Could you check a few things on this model? Use its own coordinates, in mm. Round coordinates to 2 decimals unless told otherwise and drop trailing zeros. Loops run counter-clockwise (first coordinate to the right, second up) from the corner with the lowest first, then second, coordinate; pieces in that order, holes last. Notation, with made-up numbers: (-14, 80.25) -> (15, 80.25) arc R23 cw to (15, 91.25) -> close; hole circle Ø4 at (28, 76.25). An arc over 180 degrees is marked (long way). Use CSV: the item, a comma, the result in double quotes. Start each with the question number.
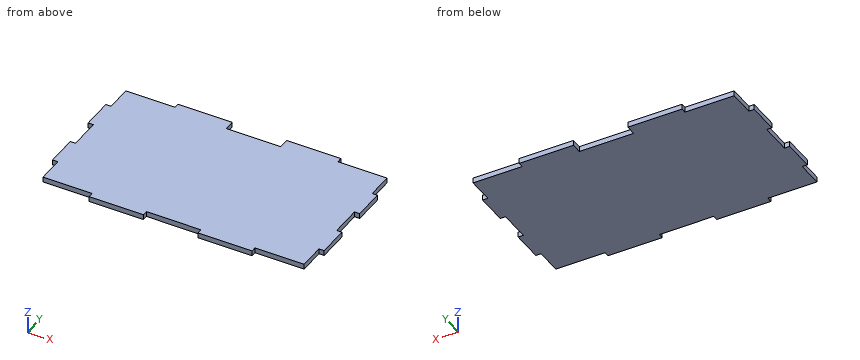
```python
from build123d import *

# Parameters (mm, degrees)
SALIENTE_EXTRUIR1_DEPTH = 5
CROQUIS2_W              = 52
CROQUIS2_H              = 5
CORTAR_EXTRUIR1_DEPTH   = 10


with BuildPart() as part:
    # Croquis1 → Saliente-Extruir1 (new body)
    with BuildSketch(Plane.XY):
        Polygon((52, 0), (104, 0), (104, 5), (156, 5), (156, 0), (208, 0), (208, 5), (255, 5), (255, 30), (260, 30), (260, 60), (255, 60), (255, 90), (260, 90), (260, 120), (255, 120), (255, 145), (208, 145), (208, 150), (156, 150), (156, 145), (104, 145), (104, 150), (52, 150), (52, 145), (5, 145), (5, 120), (0, 120), (0, 90), (5, 90), (5, 60), (0, 60), (0, 30), (5, 30), (5, 5), (52, 5), align=None)
    extrude(amount=SALIENTE_EXTRUIR1_DEPTH)

    # Croquis2 → Cortar-Extruir1 (cut)
    with BuildSketch(Plane.XY.offset(5)):
        with Locations((130, 142.5)):
            Rectangle(CROQUIS2_W, CROQUIS2_H)
    extrude(amount=-CORTAR_EXTRUIR1_DEPTH, mode=Mode.SUBTRACT)


solid = part.part
```
1. Will these pins go through, and if not, where does the flat tip stop? pin 1 (1.5 mm diameter, centred on x = 258, z = 3, fed in from +Y); pin 2 (2 mm diameter, centred on x = 145, y = 96, fed in from -Z); pin 3 (1.5 mm diameter, centred on x = 134.5, z = 2, fed in from +Y); pin 4 (2.5 mm diameter, centred on y = 2.5, z = 2, fed in from +X).
2. If I drill on L1, parallel to X at y = 143, z = 1.95; L2, parallel to Y at x = 140, z = 3.1; L3, parallel to X at y = 12, z = 4.6, over which ranges is the centre line in solid material (lowest first)?
3. Suppose I cut it at B-B (y = 16.5). List the corners of the cut face in (x, z) for me, then the cut area to 3 significant figures.
4. Suppose I cut it at A-A (x = 43). List the corners of the cut face in (y, z) for me, then the cut area to 3 significant figures.
Geometry check:
1,pin 1,"stops at y = 120"
1,pin 2,"stops at z = 0"
1,pin 3,"stops at y = 140"
1,pin 4,"stops at x = 208"
2,L1,"x = 5 to 104, 156 to 255"
2,L2,"y = 5 to 140"
2,L3,"x = 5 to 255"
3,outline,"(5, 0) -> (255, 0) -> (255, 5) -> (5, 5) -> close"
3,area,"1,250 mm²"
4,outline,"(5, 0) -> (145, 0) -> (145, 5) -> (5, 5) -> close"
4,area,"700 mm²"
